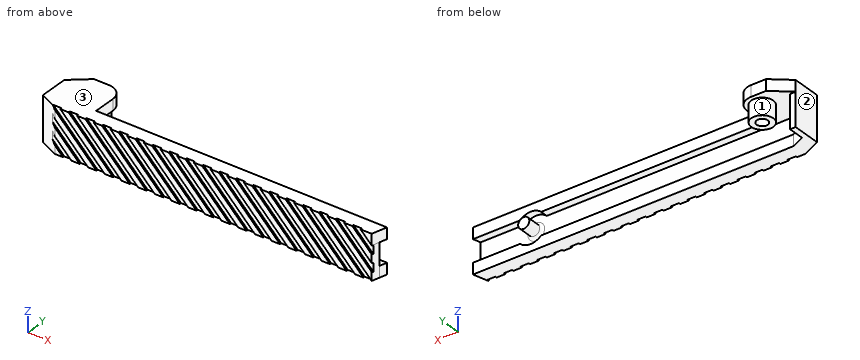
```python
from build123d import *

# Parameters (mm, degrees)
SKETCH1_R           = 1.975
BOSS_EXTRUDE1_DEPTH = 3
SKETCH2_R           = 1
CUT_EXTRUDE1_DEPTH  = 4
BOSS_EXTRUDE3_DEPTH = 2
SKETCH4_W           = 1
SKETCH4_H           = 5.097660252
BOSS_EXTRUDE5_DEPTH = 6
BOSS_EXTRUDE6_DEPTH = 6
BOSS_EXTRUDE7_DEPTH = 2
SKETCH8_R           = 1
BOSS_EXTRUDE8_DEPTH = 3
SKETCH9_R           = 2.75
SKETCH9_R_2         = 1
CUT_EXTRUDE2_DEPTH  = 3
FILLET1_R           = 0.5
CUT_EXTRUDE5_DEPTH  = 0.3


with BuildPart() as part:
    # Sketch1 → Boss-Extrude1 (new body)
    with BuildSketch(Plane.XY):
        Circle(SKETCH1_R)
    extrude(amount=BOSS_EXTRUDE1_DEPTH)

    # Sketch2 → Cut-Extrude1 (cut, through all)
    with BuildSketch(Plane.XY.offset(3)):
        Circle(SKETCH2_R)
    extrude(amount=-CUT_EXTRUDE1_DEPTH, mode=Mode.SUBTRACT)

    # Sketch3 → Boss-Extrude3 (add)
    with BuildSketch(Plane.XY.offset(3)):
        with BuildLine():
            Line((2.696329955, 0.027323162), (2.69646839, -3.972676835))
            Line((2.69646839, -3.972676835), (55, -3.972676835))
            Line((55, -3.972676835), (54.277483472, -6.669145226))
            Line((54.277483472, -6.669145226), (0, -6.669145226))
            Line((0, -6.669145226), (-2.69646839, -6.669145226))
            Line((-2.69646839, -6.669145226), (-5.965910349, -5.144579403))
            Line((-5.965910349, -5.144579403), (-5.965910349, -0.046919151))
            Line((-5.965910349, -0.046919151), (-2.69646839, 2.69646839))
            Line((-2.69646839, 2.69646839), (0, 2.69646839))
            ThreePointArc((0, 2.69646839), (1.897006291, 1.916326932), (2.696329955, 0.027323162))
        make_face()
    extrude(amount=BOSS_EXTRUDE3_DEPTH)

    # Sketch4 → Boss-Extrude5 (add)
    with BuildSketch(Plane(origin=(0, 0, 3), x_dir=(-1, 0, 0), z_dir=(0, 0, -1))):
        with Locations((5.465910349, -2.595749277)):
            Rectangle(SKETCH4_W, SKETCH4_H)
    extrude(amount=BOSS_EXTRUDE5_DEPTH)

    # Sketch5 → Boss-Extrude6 (add)
    with BuildSketch(Plane(origin=(0, 0, 3), x_dir=(-1, 0, 0), z_dir=(0, 0, -1))):
        Polygon((-54.638741736, -5.320911031), (2.690099823, -5.320911031), (4.965910349, -4.259683154), (4.965910349, -5.144579403), (5.965910349, -5.144579403), (2.69646839, -6.669145226), (-54.277483472, -6.669145226), align=None)
    extrude(amount=BOSS_EXTRUDE6_DEPTH)

    # Sketch6 → Boss-Extrude7 (add)
    with BuildSketch(Plane(origin=(0, 0, -3), x_dir=(-1, 0, 0), z_dir=(0, 0, -1))):
        Polygon((-54.638741736, -5.320911031), (-55, -3.972676835), (2.620283863, -3.972676835), (4.965910349, -2.878893242), (4.965910349, -4.259683154), (2.690099823, -5.320911031), align=None)
    extrude(amount=-BOSS_EXTRUDE7_DEPTH)

    # Sketch8 → Boss-Extrude8 (add)
    with BuildSketch(Plane(origin=(0, -5.320911031, 0), x_dir=(1, 0, 0), z_dir=(0, 1, 0))):
        with Locations((44.638741736, -1)):
            Circle(SKETCH8_R)
    extrude(amount=BOSS_EXTRUDE8_DEPTH)

    # Sketch9 → Cut-Extrude2 (cut)
    with BuildSketch(Plane(origin=(0, -5.320911031, 0), x_dir=(1, 0, 0), z_dir=(0, 1, 0))):
        with Locations((44.638741736, -1)):
            Circle(SKETCH9_R)
        with Locations((44.638741736, -1)):
            Circle(SKETCH9_R_2, mode=Mode.SUBTRACT)
    extrude(amount=CUT_EXTRUDE2_DEPTH, mode=Mode.SUBTRACT)

    # Fillet1
    fillet1_edges = [part.edges().sort_by_distance(p)[0] for p in [
        (43.638741736, -5.320911031, 1),
    ]]
    fillet(fillet1_edges, radius=FILLET1_R)

    # Sketch10 → Cut-Extrude5 (cut)
    with BuildSketch(Plane.XZ.offset(6.669145226)):
        Polygon((54.277483472, -3), (46.277483472, 5), (44.777483472, 5), (52.777483472, -3), align=None)
        Polygon((49.777483472, -3), (51.277483472, -3), (43.277483472, 5), (41.777483472, 5), align=None)
        Polygon((46.777483472, -3), (48.277483472, -3), (40.277483472, 5), (38.777483472, 5), align=None)
        Polygon((43.777483472, -3), (45.277483472, -3), (37.277483472, 5), (35.777483472, 5), align=None)
        Polygon((40.777483472, -3), (42.277483472, -3), (34.277483472, 5), (32.777483472, 5), align=None)
        Polygon((37.777483472, -3), (39.277483472, -3), (31.277483472, 5), (29.777483472, 5), align=None)
        Polygon((34.777483472, -3), (36.277483472, -3), (28.277483472, 5), (26.777483472, 5), align=None)
        Polygon((31.777483472, -3), (33.277483472, -3), (25.277483472, 5), (23.777483472, 5), align=None)
        Polygon((28.777483472, -3), (30.277483472, -3), (22.277483472, 5), (20.777483472, 5), align=None)
        Polygon((25.777483472, -3), (27.277483472, -3), (19.277483472, 5), (17.777483472, 5), align=None)
        Polygon((22.777483472, -3), (24.277483472, -3), (16.277483472, 5), (14.777483472, 5), align=None)
        Polygon((19.777483472, -3), (21.277483472, -3), (13.277483472, 5), (11.777483472, 5), align=None)
        Polygon((16.777483472, -3), (18.277483472, -3), (10.277483472, 5), (8.777483472, 5), align=None)
        Polygon((13.777483472, -3), (15.277483472, -3), (7.277483472, 5), (5.777483472, 5), align=None)
        Polygon((10.777483472, -3), (12.277483472, -3), (4.277483472, 5), (2.777483472, 5), align=None)
        Polygon((7.777483472, -3), (9.277483472, -3), (1.277483472, 5), (-0.222516528, 5), align=None)
        Polygon((4.777483472, -3), (6.277483472, -3), (-1.722516528, 5), (-3.222516528, 5), align=None)
        Polygon((1.777483472, -3), (3.277483472, -3), (-4.722516528, 5), (-6.222516528, 5), align=None)
        Polygon((-1.222516528, -3), (0.277483472, -3), (-7.722516528, 5), (-9.222516528, 5), align=None)
        Polygon((55.777483472, -3), (57.277483472, -3), (49.277483472, 5), (47.777483472, 5), align=None)
        Polygon((58.777483472, -3), (60.277483472, -3), (52.277483472, 5), (50.777483472, 5), align=None)
    extrude(amount=-CUT_EXTRUDE5_DEPTH, mode=Mode.SUBTRACT)


solid = part.part
```
Verification items for the finished model (mm, model axes). Face numbers are marked on the shaded views. Give positions to 0.01 mm unless a question says otherwise; leave off trailing zeros. One line per item, written item: value.
(1) Draft check along X on the marked faces 1, 2 and 3. Enter one of: pulls with the +X half, pulls with the -X half, needs draft (parallel to the pull), parting line crosses it, or undercut.
Final values:
face 1: undercut
face 2: pulls with the -X half
face 3: needs draft
(2) Scan lines: line 1 along Y through (x, z) = (0, 2) (3 decimals); line 2 along Y through (x, z) = (0, 1.65) (3 decimals); line 3 along Z through (x, y) = (6.5, -5.25). Record each from-to range of solid material in increasing order. Write a range as [from, to].
Final values:
line 1: [-6.369, -5.321], [-1.975, -1], [1, 1.975]
line 2: [-6.669, -5.321], [-1.975, -1], [1, 1.975]
line 3: [-3, -1], [3, 5]
(3) Gauge pin test, flat ends, axial feed: pin 1 (2 mm diameter, centred on x = 38.5, z = 3, fed in from +Y); pin 2 (1.6 mm diameter, centred on x = 39, z = 1, fed in from +Y). Record the tip position at first contact, or that the pin passes through.
Final values:
pin 1: y = -3.97
pin 2: y = -5.32
